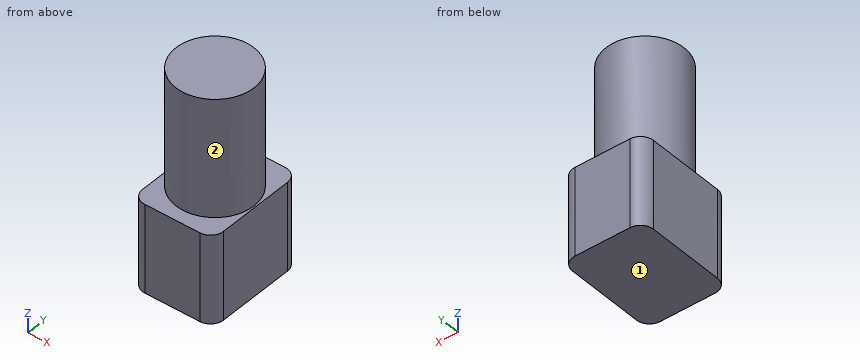
from build123d import *

# Parameters (mm, degrees)
F0_R     = 9.525
F1_DEPTH = 28.7274
F2_W     = 19.80688
F2_H     = 25.4
F3_DEPTH = 21.59
F4_R     = 3.175


with BuildPart() as f1:
    # F0 (on Top) → F1 (new body)
    with BuildSketch(Plane.XY):
        Circle(F0_R)
    extrude(amount=F1_DEPTH)

    # F2 (on face) → F3 (join)
    with BuildSketch(Plane(origin=(0, 0, 0), x_dir=(1, 0, 0), z_dir=(0, 0, -1))):
        Rectangle(F2_W, F2_H)
    extrude(amount=F3_DEPTH)

    # F4
    f4_edges = [f1.edges().sort_by_distance(p)[0] for p in [
        (9.90344, -12.7, -10.795),
        (-9.90344, -12.7, -10.795),
        (9.90344, 12.7, -10.795),
        (-9.90344, 12.7, -10.795),
    ]]
    fillet(f4_edges, radius=F4_R)


solid = f1.part
The listing builds one solid part. Answer for the finished solid, in the listing's coordinates (mm). Face numbers are marked on the shaded views. A direction names the side the tool comes from. Round coordinates to 2 decimals unless told otherwise and drop trailing zeros. Write each loop counter-clockwise with the first axis right and the second up, starting at its lowest first coordinate (ties: lowest second). Pieces come first, ordered by that corner, then holes. Notation, with made-up numbers: (-13.75, 79) - (-9.75, 79) arc R11 ccw to (-9.75, 88) - close; hole circle Ø6 at (16, 13.5). An arc over 180 degrees is marked (long way). Use a Markdown table: item, result. Add a question column.
1. The part is cut by section A-A (z = -17). Write down the section's boundary in (x, y) (3 decimals), and give its area (3 significant figures).
2. A tool of negligible diameter and unlimited length cuts with its end or side. For the marked faces 1 and 2, from which of +Z, -Z, +X, -X, +Y, -Y can it reach the whole face along a straight path? Write none if from no direction.
3. Consider line 1 (Z direction, x = 6.75, y = 9.5); line 2 (Y direction, x = 1.5, z = 15.5); line 3 (Y direction, x = -4.5, z = 19). Determine where each line is inside the solid, lowest interval first.
4. The part is cut by section B-B (x = 0). Write down the section's boundary in (y, z) (3 decimals).
5. The part is cut by section C-C (y = 11). Write down the section's boundary in (x, z), and give its area (3 significant figures).
6. The part is cut by section D-D (z = 22). Write down the section's boundary in (x, y) (3 decimals).
7. Flat-ended cylindrical pins translate along their axes: P1, Ø8, axis at x = 5, z = 8.5, coming from the -Y side; P2, Ø5, axis at x = -7.5, z = -16.5, coming from the +Y side; P3, Ø1.5, axis at x = 5, z = 22, coming from the +Y side. Find the tip coordinate at first contact, or state that the pin passes through.
Reported:
| question | item | result |
|---|---|---|
| 1 | outline | (-9.903, -9.525) arc R3.175 ccw to (-6.728, -12.7) - (6.728, -12.7) arc R3.175 ccw to (9.903, -9.525) - (9.903, 9.525) arc R3.175 ccw to (6.728, 12.7) - (-6.728, 12.7) arc R3.175 ccw to (-9.903, 9.525) - close |
| 1 | area | 494 mm^2 |
| 2 | face 1 | -Z, +X, -X, +Y, -Y |
| 2 | face 2 | +Z |
| 3 | line 1 | -21.59 to 0 |
| 3 | line 2 | -9.41 to 9.41 |
| 3 | line 3 | -8.39 to 8.39 |
| 4 | outline | (-12.7, -21.59) - (12.7, -21.59) - (12.7, 0) - (9.525, 0) - (9.525, 28.727) - (-9.525, 28.727) - (-9.525, 0) - (-12.7, 0) - close |
| 5 | outline | (-9.54, -21.59) - (9.54, -21.59) - (9.54, 0) - (-9.54, 0) - close |
| 5 | area | 412 mm^2 |
| 6 | outline | circle Ø19.05 at (0, 0) |
| 7 | P1 | y = -9.47 |
| 7 | P2 | y = 12.7 |
| 7 | P3 | y = 8.52 |
